Answer from the drawing. Dimensions are ordinates in mm from the lowest x, y and z of the part. Give positions to 0.01 mm unless a question says otherwise; leave off trailing zeros. Write each loop counter-clockwise with the first axis right and the second up, starting at its lowest first coordinate (ties: lowest second). Pieces come first, ordered by that corner, then holes. Notation, with made-up numbers: M 35.25,9 L 55.25,9 A17 cw 55.25,19 Z; hole C -33,41 d3. An arc over 180 degrees is marked long. Put each result on its own line as item: value.
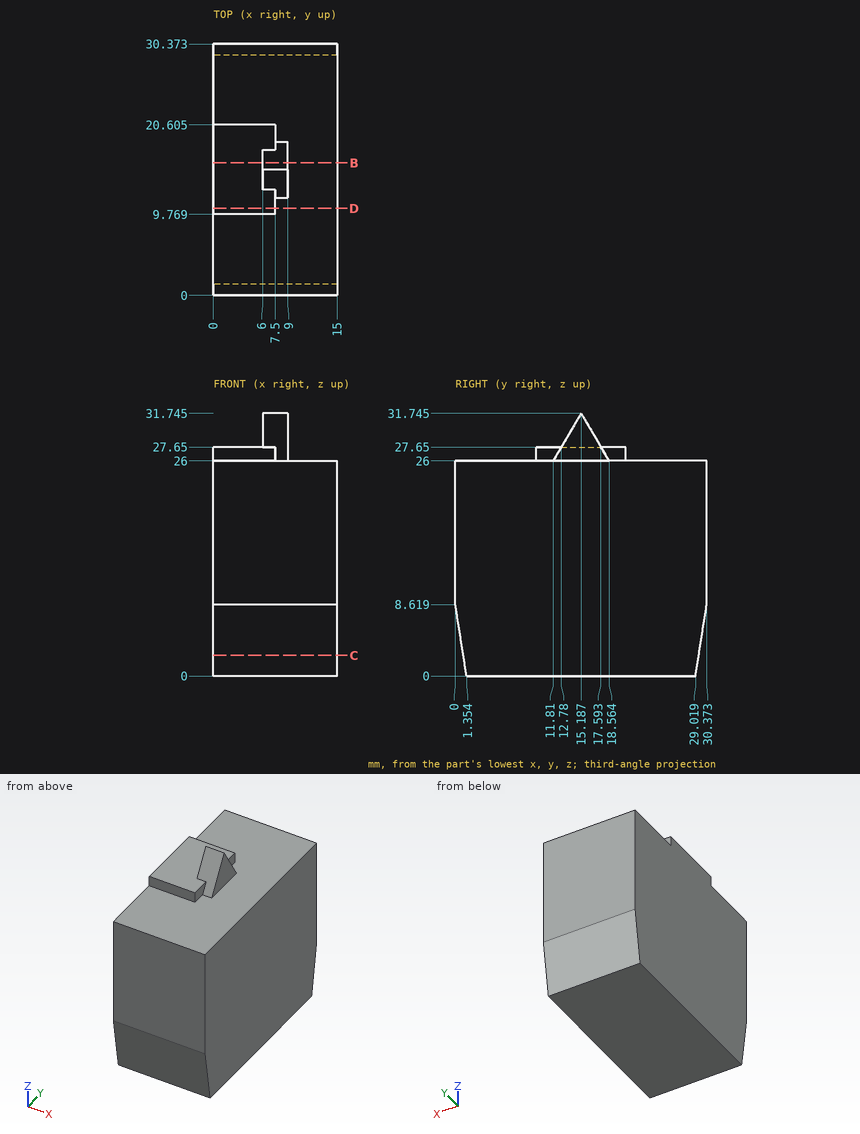
(1) Section C-C on z = 2.5 is taken. Determine the outline of the cut face in (x, y).
Result:
outline: M 0,0.96 L 15,0.96 L 15,29.41 L 0,29.41 Z
(2) Section D-D on y = 10.5 is taken. Determine the outline of the cut face in (x, z).
Result:
outline: M 0,0 L 15,0 L 15,26 L 7.5,26 L 7.5,27.65 L 0,27.65 Z
(3) Straight lines are drawn through the part: line 1 along Y through (x, z) = (6, 26.5) (1 decimal); line 2 along Z through (x, y) = (13, 26.5); line 3 along Z through (x, y) = (1, 17). For each, find the intervals that lie inside material, in ascending order. Write a range as from..to.
Result:
line 1: y = 9.8..20.6
line 2: z = 0..26
line 3: z = 0..27.65
(4) Given pin 1 Ø1.8 at (y, z) = (19.5, 27) entering from +X; pin 2 Ø4 at (x, y) = (2.5, 17) entering from +Z; pin 3 Ø1 at (x, z) = (13, 4) entering from +Y, each flat-ended and moving along its own axis, determine where each tip first touches the part or whether it passes through.
Result:
pin 1: stops at x = 7.5
pin 2: stops at z = 27.65
pin 3: stops at y = 29.73
(5) Section B-B on y = 16 is taken. Determine the outline of the cut face in (x, z), and give its area (3 significant figures).
Result:
outline: M 0,0 L 15,0 L 15,26 L 9,26 L 9,30.36 L 6,30.36 L 6,27.65 L 0,27.65 Z
area: 413 mm²
